Could you check a few things on this model? Use its own coordinates, in mm. A direction names the side the tool comes from. Give positions to 0.01 mm unless a question says otherwise; leave off trailing zeros. Loops run counter-clockwise (first coordinate to the right, second up) from the corner with the lowest first, then second, coordinate; pieces in that order, holes last.
1. Imagine slicing it at A-A (x = 2). List the corners of the cut face in (y, z) for me, plus the area to 3 significant figures.
2. For faces 4 (the flat face through (12.552, -22, 9)), 5 (the flat face through (-38, 10, 9)), 6 (the flat face through (-20, -5, 9)), 7 (the flat face through (35, 15, 9)), 8 (the flat face through (-22.448, -15, 9)), which set-ups out of +Z, -Z, +X, -X, +Y, -Y let a thin tool reach every point of the face, with its end or its side?
3. Thinking about a two-plate mould opening in Y: for faces 1 (the flat face through (8.3, -25, 2.6)), 2 (the flat face through (-1, -16, 3)), 3 (the flat face through (-35, 15, 9)), which applies, +Y half, -Y half, draft (parallel to the pull), parting line (faces both ways), or undercut?
4. Imagine slicing it at B-B (y = -1). List the corners of the cut face in (x, z) for me.
5. Imagine slicing it at D-D (y = 18.5). List the corners of the cut face in (x, z) for me.
6. For P1, Ø6.5, axis at x = -26, z = 7, coming from the -Y side; P2, Ø6.5, axis at y = -10, z = 7.5, coming from the -X side; P3, Ø15, axis at x = 13.5, y = -2.5, coming from the +Z side; P4, Ø4, axis at x = 0, y = -17, coming from the +Z side, each with a flat end and sliding along its axis, tell me the tip position at first contact or that it passes through.
7. Imagine slicing it at C-C (z = 5.5). List the corners of the cut face in (x, y) for me, plus the area to 3 significant figures.
8. I need wall thicknesses on line 1 along Y through (x, z) = (19, 7.25); line 2 along X through (y, z) = (-10, 6.75); line 3 along X through (y, z) = (-10, 2.75). Which ranges of each line are inside material? Lowest first, please.
```python
from build123d import *

# Parameters (mm, degrees)
F0_W     = 80
F0_H     = 50
F1_DEPTH = 3
F3_DEPTH = 16
F5_DEPTH = 25


with BuildPart() as f1:
    # F0 (on Top) → F1 (new body)
    with BuildSketch(Plane.XY):
        Rectangle(F0_W, F0_H)
    extrude(amount=F1_DEPTH)

    # F2 (on Top) → F3 (join)
    with BuildSketch(Plane.XY):
        Polygon((-35, 20), (0, 20), (0, 25), (-40, 25), (-40, 10), (-35, 10), align=None)
        Polygon((40, 25), (10, 25), (10, 20), (35, 20), (35, 10), (40, 10), align=None)
        Polygon((40, -25), (40, -5), (32.552384, -5), (32.552384, -20), (12.552384, -20), (12.552384, -25), align=None)
        Polygon((-22.447616, -25), (-17.447616, -25), (-17.447616, -5), (-22.447616, -5), (-22.447616, -20), align=None)
    extrude(amount=F3_DEPTH)


with BuildPart() as f5:
    # F4 (on Top) → F5 (new body)
    with BuildSketch(Plane.XY):
        Polygon((-30, 0), (-10, 0), (-10, -15), (25, -15), (25, 15), (-30, 15), align=None)
    extrude(amount=F5_DEPTH)


with BuildPart() as f1_1:
    add(f1.part)

    # F6: cut F5
    add(f5.part, mode=Mode.SUBTRACT)


solid = f1_1.part
```
Derived:
1. outline: (-25, 0) - (-15, 0) - (-15, 3) - (-25, 3) - close; (15, 0) - (25, 0) - (25, 3) - (15, 3) - close
1. area: 60.0 mm2
2. face 4: +Z, -Y
2. face 5: +Z, +X, -X, -Y
2. face 6: +Z, +X, -X
2. face 7: +Z
2. face 8: +Z, -X, -Y
3. face 1: -Y half
3. face 2: undercut
3. face 3: draft
4. outline: (-40, 0) - (-10, 0) - (-10, 3) - (-40, 3) - close; (25, 0) - (40, 0) - (40, 3) - (25, 3) - close
5. outline: (-40, 0) - (40, 0) - (40, 16) - (35, 16) - (35, 3) - (-35, 3) - (-35, 16) - (-40, 16) - close
6. P1: stops at y = 20
6. P2: stops at x = -22.45
6. P3: passes through
6. P4: stops at z = 3
7. outline: (-40, 10) - (-35, 10) - (-35, 20) - (0, 20) - (0, 25) - (-40, 25) - close; (-22.45, -25) - (-17.45, -25) - (-17.45, -5) - (-22.45, -5) - close; (10, 20) - (35, 20) - (35, 10) - (40, 10) - (40, 25) - (10, 25) - close; (12.55, -25) - (40, -25) - (40, -5) - (32.55, -5) - (32.55, -20) - (12.55, -20) - close
7. area: 799 mm2
8. line 1: y = -25 to -20, 20 to 25
8. line 2: x = -22.45 to -17.45, 32.55 to 40
8. line 3: x = -40 to -10, 25 to 40
